Design review of the part built by this model. Coordinates are the model's own, in mm. Face numbers are marked on the shaded views. A direction names the side the tool comes from. Give positions to 0.01 mm unless a question says otherwise; leave off trailing zeros. Loops run counter-clockwise (first coordinate to the right, second up) from the corner with the lowest first, then second, coordinate; pieces in that order, holes last. Notation, with made-up numbers: (-34.75, -1) -> (10.25, -1) arc R29 cw to (10.25, 38) -> close; hole circle Ø6 at (-38.75, 65). An arc over 180 degrees is marked (long way). Answer as CSV lines item,"result".
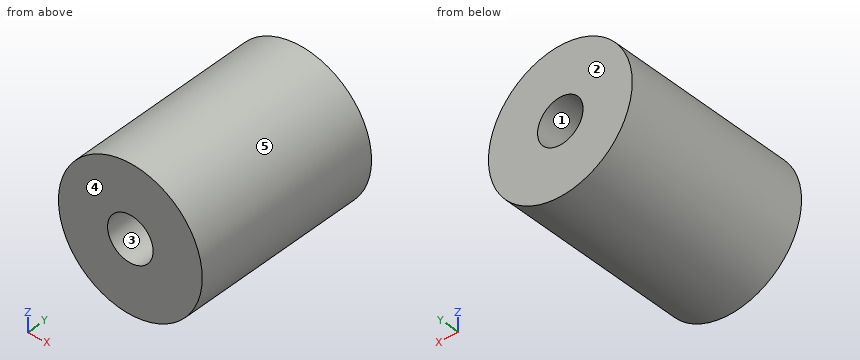
from build123d import *

# Parameters (mm, degrees)
SKETCH1_R           = 7.5
BOSS_EXTRUDE1_DEPTH = 10
SKETCH2_R           = 2.375
CUT_EXTRUDE1_DEPTH  = 9
SKETCH3_R           = 2.375
CUT_EXTRUDE2_DEPTH  = 9


with BuildPart() as part:
    # Sketch1 → Boss-Extrude1 (new body, symmetric)
    with BuildSketch(Plane(origin=(0, 0, 0), x_dir=(1, 0, 0), z_dir=(0, 1, 0))):
        Circle(SKETCH1_R)
    extrude(amount=BOSS_EXTRUDE1_DEPTH, both=True)

    # Sketch2 → Cut-Extrude1 (cut)
    with BuildSketch(Plane(origin=(0, 10, 0), x_dir=(1, 0, 0), z_dir=(0, 1, 0))):
        Circle(SKETCH2_R)
    extrude(amount=-CUT_EXTRUDE1_DEPTH, mode=Mode.SUBTRACT)

    # Sketch3 → Cut-Extrude2 (cut)
    with BuildSketch(Plane.XZ.offset(10)):
        Circle(SKETCH3_R)
    extrude(amount=-CUT_EXTRUDE2_DEPTH, mode=Mode.SUBTRACT)


solid = part.part
Q1. Clearance check with flat-ended pins moving along their axes: pin 1 Ø5 at (x, z) = (-1, -1) entering from +Y; pin 2 Ø6 at (y, z) = (-2, -4) entering from -X; pin 3 Ø5 at (x, y) = (3.5, 3.5) entering from +Z; pin 4 Ø1 at (x, y) = (-6, 7) entering from +Z. State where each tip first meets the part, or that it passes through.
Filled sheet:
pin 1,"stops at y = 10"
pin 2,"stops at x = -7.43"
pin 3,"stops at z = 7.43"
pin 4,"stops at z = 5.1"
Q2. We need section D-D, the plane y = -6.25. State the section outline as (x, z) points (3 decimals).
Filled sheet:
outline,"circle Ø15 at (0, 0); hole circle Ø4.75 at (0, 0)"
Q3. We need section B-B, the plane z = 0. State the section outline as (x, y) points (3 decimals), and give its area (4 significant figures).
Filled sheet:
outline,"(-7.5, -10) -> (-2.375, -10) -> (-2.375, -1) -> (2.375, -1) -> (2.375, -10) -> (7.5, -10) -> (7.5, 10) -> (2.375, 10) -> (2.375, 1) -> (-2.375, 1) -> (-2.375, 10) -> (-7.5, 10) -> close"
area,"214.5 mm^2"
Q4. We need section A-A, the plane x = 0. State the section outline as (y, z) points (3 decimals), and give its area (4 significant figures).
Filled sheet:
outline,"(-10, -7.5) -> (10, -7.5) -> (10, -2.375) -> (1, -2.375) -> (1, 2.375) -> (10, 2.375) -> (10, 7.5) -> (-10, 7.5) -> (-10, 2.375) -> (-1, 2.375) -> (-1, -2.375) -> (-10, -2.375) -> close"
area,"214.5 mm^2"
Q5. The part is to be moulded in two halves that separate along Z. For the marked faces 3, 4 and 5, say which applies: pulls with the +Z half, pulls with the -Z half, needs draft (parallel to the pull), parting line crosses it, or undercut.
Filled sheet:
face 3,"undercut"
face 4,"needs draft"
face 5,"parting line crosses it"
Q6. To check wall thickness, follow probe 1 along X at (y, z) = (4.25, 0) (3 decimals); probe 2 along Y at (x, z) = (-1.25, 0.75). State the ranges of each line that lie inside material, in increasing order. Write a range as from..to.
Filled sheet:
probe 1,"x = -7.5..-2.375, 2.375..7.5"
probe 2,"y = -1..1"
Q7. For the marked faces 1 and 2, list the 3-axis set-ups (+Z, -Z, +X, -X, +Y, -Y) from which the entire face can be reached by the end or side of a thin tool; tool diameter is ignored.
Filled sheet:
face 1,"+Y"
face 2,"+Z, -Z, +X, -X, +Y"
Q8. We need section C-C, the plane y = -0.25. State the section outline as (x, z) points, and give its area (3 significant figures).
Filled sheet:
outline,"circle Ø15 at (0, 0)"
area,"177 mm^2"
